Geometry check sheet. Reference: the model listing, model coordinates, mm. A direction names the side the tool comes from. Coordinates: 2 decimals unless noted, no trailing zeros. Loops run counter-clockwise (first coordinate to the right, second up) from the corner with the lowest first, then second, coordinate; pieces in that order, holes last.
from build123d import *

# Parameters (mm, degrees)
SKETCH1_W           = 115
SKETCH1_H           = 65
BOSS_EXTRUDE1_DEPTH = 5
SKETCH2_R           = 1.5
CUT_EXTRUDE1_DEPTH  = 67.238206497
CHAMFER1_SIZE       = 3
CHAMFER1_SIZE_2     = 7
FILLET1_R           = 7
SKETCH3_W           = 101
SKETCH3_H           = 65
BOSS_EXTRUDE2_DEPTH = 13.8
FILLET2_R           = 3.5
SKETCH4_W           = 26
SKETCH4_H           = 8
CUT_EXTRUDE2_DEPTH  = 6.6
SKETCH5_W           = 54.5
SKETCH5_H           = 8
CUT_EXTRUDE3_DEPTH  = 6.6


# Some blends are built 0.0001 mm under size
with BuildPart() as part:
    # Sketch1 → Boss-Extrude1 (new body)
    with BuildSketch(Plane(origin=(0, 0, 0), x_dir=(1, 0, 0), z_dir=(0, 1, 0))):
        Rectangle(SKETCH1_W, SKETCH1_H)
    extrude(amount=BOSS_EXTRUDE1_DEPTH)

    # Sketch2 → Cut-Extrude1 (cut, through all)
    with BuildSketch(Plane(origin=(0, 5, 0), x_dir=(1, 0, 0), z_dir=(0, 1, 0))):
        with Locations(Location((53.5, 20, 0), (0, 0, 270))):
            Circle(SKETCH2_R)
        with Locations(Location((53.5, -20, 0), (0, 0, 270))):
            Circle(SKETCH2_R)
    cut_extrude1 = extrude(amount=-CUT_EXTRUDE1_DEPTH, mode=Mode.SUBTRACT)

    # Mirror16: Cut-Extrude1 across plane
    add(cut_extrude1.mirror(Plane(origin=(0, 0, 0), x_dir=(0, 0, 1), z_dir=(1, 0, 0))), mode=Mode.SUBTRACT)

    # Chamfer1
    # the kernel refuses this chamfer: 7, 3 mm, written as the material it takes off along each edge
    with BuildSketch(Plane(origin=(-57.5, 5, -50.645496776), x_dir=(-0.08246287738523231, -0.9965941369752023, 0), z_dir=(0, 0, 1)), Plane(origin=(57.5, 5, 50.645496776), x_dir=(0.08246287738523231, -0.9965941369752023, 0), z_dir=(0, 0, -1))) as chamfer1_piece_1:
        Polygon((CHAMFER1_SIZE * 0.996594136975, CHAMFER1_SIZE * 0.0824628773852), (-CHAMFER1_SIZE_2 * 0.0824628773852, CHAMFER1_SIZE_2 * 0.996594136975), (0, 0), align=None)
    extrude(amount=101.290993551, mode=Mode.SUBTRACT)

    # Fillet1
    fillet1_edges = [part.edges().sort_by_distance(p)[0] for p in [
        (57.5, 1, -32.5),
        (57.5, 1, 32.5),
        (-57.5, 1, -32.5),
        (-57.5, 1, 32.5),
    ]]
    fillet(fillet1_edges, radius=FILLET1_R - 0.0001)  # a hair under: the kernel refuses the full size

    # Sketch3 → Boss-Extrude2 (add)
    with BuildSketch(Plane(origin=(0, 5, 0), x_dir=(1, 0, 0), z_dir=(0, 1, 0))):
        Rectangle(SKETCH3_W, SKETCH3_H)
    extrude(amount=BOSS_EXTRUDE2_DEPTH)

    # Fillet2
    fillet2_edges = [part.edges().sort_by_distance(p)[0] for p in [
        (0, 18.8, 32.5),
        (-50.5, 11.9, 32.5),
        (-50.5, 18.8, 0),
        (-50.5, 11.9, -32.5),
        (0, 18.8, -32.5),
        (50.5, 11.9, -32.5),
        (50.5, 18.8, 0),
        (50.5, 11.9, 32.5),
    ]]
    fillet(fillet2_edges, radius=FILLET2_R)

    # Sketch4 → Cut-Extrude2 (cut)
    with BuildSketch(Plane.ZY.offset(50.5)):
        with Locations((-0.5, 9)):
            Rectangle(SKETCH4_W, SKETCH4_H)
    extrude(amount=-CUT_EXTRUDE2_DEPTH, mode=Mode.SUBTRACT)

    # Sketch5 → Cut-Extrude3 (cut)
    with BuildSketch(Plane(origin=(50.5, 0, 0), x_dir=(0, 0, -1), z_dir=(1, 0, 0))):
        with Locations((-0.75, 9)):
            Rectangle(SKETCH5_W, SKETCH5_H)
    extrude(amount=-CUT_EXTRUDE3_DEPTH, mode=Mode.SUBTRACT)


solid = part.part
1) Access from +Z, -Z, +X, -X, +Y, -Y to the whole of each face (thin tool, end or side, straight path). Record for faces 4 (the cylindrical face through (52, 2, 20)), 5 (the cylindrical face through (49.45, 10.22, -31.5)), 6 (the cylindrical face through (-49.5, 10.22, 31.45)), 7 (the cylindrical face through (-49.5, 10.22, -31.45)), 8 (the flat face through (-43.9, 9, -1)).
Data:
face 4: +Y, -Y
face 5: -Z, +X, +Y
face 6: +Z, -X, +Y
face 7: -Z, -X, +Y
face 8: -X
2) Section check C-C on y = 10.25. Record the cut outline in (x, z).
Data:
outline: (-50.5, -29) arc R3.5 ccw to (-47, -32.5) - (47, -32.5) arc R3.5 ccw to (50.5, -29) - (50.5, -26.5) - (43.9, -26.5) - (43.9, 28) - (50.5, 28) - (50.5, 29) arc R3.5 ccw to (47, 32.5) - (-47, 32.5) arc R3.5 ccw to (-50.5, 29) - (-50.5, 12.5) - (-43.9, 12.5) - (-43.9, -13.5) - (-50.5, -13.5) - close
3) Mould release check, pull along Z, two halves, no side actions. Record for faces 1 (the flat face through (-1, 8, -32.5)), 2 (the cylindrical face through (52, 2, -20)), 3 (the cylindrical face through (-54.58, 1.42, 31.19)): +Z half, -Z half, draft (parallel to the pull), parting line (faces both ways), or undercut.
Data:
face 1: -Z half
face 2: undercut
face 3: +Z half
4) Section check D-D on z = -20. Record the cut outline in (x, y).
Data:
outline: (-57.5, 0) - (-55, 0) - (-55, 3.07) - (-57.5, 2) - close; (-52, 0) - (52, 0) - (52, 4.36) - (50.5, 5) - (43.9, 5) - (43.9, 13) - (50.5, 13) - (50.5, 15.3) arc R3.5 ccw to (47, 18.8) - (-47, 18.8) arc R3.5 ccw to (-50.5, 15.3) - (-50.5, 5) - (-52, 4.36) - close; (55, 0) - (57.5, 0) - (57.5, 2) - (55, 3.07) - close
5) Section check B-B on z = -10. Record the cut outline in (x, y).
Data:
outline: (-57.5, 0) - (57.5, 0) - (57.5, 2) - (50.5, 5) - (43.9, 5) - (43.9, 13) - (50.5, 13) - (50.5, 15.3) arc R3.5 ccw to (47, 18.8) - (-47, 18.8) arc R3.5 ccw to (-50.5, 15.3) - (-50.5, 13) - (-43.9, 13) - (-43.9, 5) - (-50.5, 5) - (-57.5, 2) - close
6) Section check A-A on x = 53.5. Record the cut outline in (y, z), and give its area (3 significant figures).
Data:
outline: (0, -31.82) - (3.71, -31.82) - (3.71, -21.5) - (0, -21.5) - close; (0, -18.5) - (3.71, -18.5) - (3.71, 18.5) - (0, 18.5) - close; (0, 21.5) - (3.71, 21.5) - (3.71, 31.82) - (0, 31.82) - close
area: 214 mm2
7) Depth check by flat-ended pin: pin 1 (7.5 mm diameter, centred on x = -48, y = 10, fed in from -Z); pin 2 (1 mm diameter, centred on x = -7.5, y = 17, fed in from +Z); pin 3 (3 mm diameter, centred on y = 9, z = -2, fed in from -X); pin 4 (1.8 mm diameter, centred on x = 53.5, z = -20, fed in from +Y). Enter the tip coordinate at first touch or a pass-through.
Data:
pin 1: stops at z = -32.5
pin 2: stops at z = 32.29
pin 3: stops at x = -43.9
pin 4: passes through
8) Material ranges on probe 1 along X at (y, z) = (2.25, 20); probe 2 along X at (y, z) = (2.7, -20); probe 3 along Z at (x, y) = (-53.5, 1.05), recorded low to high.
Data:
probe 1: x = -56.92 to -55, -52 to 52, 55 to 56.92
probe 2: x = -55.87 to -55, -52 to 52, 55 to 55.87
probe 3: z = -31.82 to -21.5, -18.5 to 18.5, 21.5 to 31.82
